from build123d import *

# Parameters (mm, degrees)
SKETCH1_W                       = 18
SKETCH1_H                       = 12
EXTRUDE1_DEPTH                  = 2
SKETCH2_W                       = 1.5
SKETCH2_H                       = 0.5
EXTRUDE2_DEPTH                  = 13
EXTRUDE3_DEPTH                  = 3
MIRROR2_COPY_1_DEPTH            = 3
SKETCH4_W                       = 6.5
SKETCH4_H                       = 12
EXTRUDE4_DEPTH                  = 5
SKETCH5_W                       = 1.5
SKETCH5_H                       = 0.8
EXTRUDE5_DEPTH                  = 13
F_2_56_TAPPED_HOLE1_D           = 1.778
F_2_56_TAPPED_HOLE1_DEPTH       = 9.4488
F_2_56_TAPPED_HOLE1_CBORE_D     = 2.1844
F_2_56_TAPPED_HOLE1_CBORE_DEPTH = 5.5372
F_2_56_TAPPED_HOLE1_TIP         = 0.53416509
SKETCH7_R                       = 1.5113
EXTRUDE6_DEPTH                  = 3.0226


with BuildPart() as part:
    # Sketch1 → Extrude1 (new body)
    with BuildSketch(Plane(origin=(0, 0, 0), x_dir=(1, 0, 0), z_dir=(0, 1, 0))):
        with Locations((-9, 6)):
            Rectangle(SKETCH1_W, SKETCH1_H)
    extrude(amount=-EXTRUDE1_DEPTH)

    # Sketch2 → Extrude2 (cut, through all)
    with BuildSketch(Plane.XY):
        with Locations((-9, -1.75)):
            Rectangle(SKETCH2_W, SKETCH2_H)
    extrude(amount=-EXTRUDE2_DEPTH, mode=Mode.SUBTRACT)

    # Sketch3 → Extrude3 (cut, through all)
    with BuildSketch(Plane(origin=(0, 0, 0), x_dir=(1, 0, 0), z_dir=(0, 1, 0))):
        with BuildLine():
            Line((-16.793731354, 2.5), (-16.793731354, 3.5))
            ThreePointArc((-16.793731354, 3.5), (-15.293731354, 5), (-13.793731354, 3.5))
            Line((-13.793731354, 3.5), (-13.793731354, 2.5))
            ThreePointArc((-13.793731354, 2.5), (-15.293731354, 1), (-16.793731354, 2.5))
        make_face()
    extrude3 = extrude(amount=-EXTRUDE3_DEPTH, mode=Mode.SUBTRACT)

    # Mirror1: Extrude3 across plane
    add(extrude3.mirror(Plane(origin=(0, 0, -6), x_dir=(1, 0, 0), z_dir=(0, 0, -1))), mode=Mode.SUBTRACT)

    # Mirror2: Extrude3 across plane
    add(extrude3.mirror(Plane(origin=(-9, 0, 0), x_dir=(0, 0, 1), z_dir=(1, 0, 0))), mode=Mode.SUBTRACT)

    # Mirror2 copy 1 sketch → Mirror2 copy 1 (cut, through all)
    with BuildSketch(Plane(origin=(-18, 0, -12), x_dir=(-1, 0, 0), z_dir=(0, 1, 0))):
        with BuildLine():
            Line((-16.793731354, 2.5), (-16.793731354, 3.5))
            ThreePointArc((-16.793731354, 3.5), (-15.293731354, 5), (-13.793731354, 3.5))
            Line((-13.793731354, 3.5), (-13.793731354, 2.5))
            ThreePointArc((-13.793731354, 2.5), (-15.293731354, 1), (-16.793731354, 2.5))
        make_face()
    extrude(amount=-MIRROR2_COPY_1_DEPTH, mode=Mode.SUBTRACT)

    # Sketch4 → Extrude4 (add)
    with BuildSketch(Plane(origin=(0, 0, 0), x_dir=(1, 0, 0), z_dir=(0, 1, 0))):
        with Locations((-8.75, 6)):
            Rectangle(SKETCH4_W, SKETCH4_H)
    extrude(amount=EXTRUDE4_DEPTH)

    # Sketch5 → Extrude5 (cut, through all)
    with BuildSketch(Plane.XY):
        with Locations((-11.25, 4.6)):
            Rectangle(SKETCH5_W, SKETCH5_H)
    extrude(amount=-EXTRUDE5_DEPTH, mode=Mode.SUBTRACT)

    # #2-56 Tapped Hole1
    with Locations(Plane(origin=(-8, 5, -2.6), x_dir=(0, 0, 1), z_dir=(0, 1, 0))):
        with Locations((0, 0), (-6.8, 0)):
            CounterBoreHole(F_2_56_TAPPED_HOLE1_D / 2, F_2_56_TAPPED_HOLE1_CBORE_D / 2, F_2_56_TAPPED_HOLE1_CBORE_DEPTH, depth=F_2_56_TAPPED_HOLE1_DEPTH)
            with Locations((0, 0, -(F_2_56_TAPPED_HOLE1_DEPTH + F_2_56_TAPPED_HOLE1_TIP / 2))):  # 118° drill point
                Cone(0, F_2_56_TAPPED_HOLE1_D / 2, F_2_56_TAPPED_HOLE1_TIP, mode=Mode.SUBTRACT)

    # Sketch7 → Extrude6 (cut)
    with BuildSketch(Plane.XY):
        with Locations((-9, 0.3)):
            Circle(SKETCH7_R)
    extrude6 = extrude(amount=-EXTRUDE6_DEPTH, mode=Mode.SUBTRACT)

    # Mirror3: Extrude6 across plane
    add(extrude6.mirror(Plane(origin=(0, 0, -6), x_dir=(1, 0, 0), z_dir=(0, 0, -1))), mode=Mode.SUBTRACT)


solid = part.part
Work out the finished part from the listing and answer in its coordinate system (mm). A direction names the side the tool comes from. Coordinates: 2 decimals unless noted, no trailing zeros. Order: outer loops, then holes, each group sorted by start corner. A loop starts at its lowest first (then second) coordinate and runs counter-clockwise, first axis right, second up. Notation, with made-up numbers: (43.25, 28) - (48.25, 28) arc R13 cw to (48.25, 43) - close; hole circle Ø4 at (84, 29.25). An arc over 180 degrees is marked (long way). Put each result on its own line as item: value. Start each with the question number.
1) For a pull along Z with two mould halves and no side action, classify faces 1 (the flat face through (-10, 0, -3.023)), 2 (the cylindrical face through (-7.12, -1.28, -9.28)), 3 (the flat face through (-14, -2, -6)) as released by +Z, released by -Z, zero draft, split by the parting line, or undercut.
2) Find the intervals of material crossed by line 1 (Z direction, x = -8, y = 3.1); line 2 (X direction, y = -1.25, z = -2.6); line 3 (Z direction, x = -14, y = -0.5), in increasing order. Write a range as from..to.
3) Find section A-A (z = -6.75). Give the vertices of the cut face in (x, y), plus the area to 4 significant figures.
4) Find section C-C (z = -2.25). Give the vertices of the cut face in (x, y), plus the area to 3 significant figures.
5) Find section B-B (y = 2.25). Give the vertices of the cut face in (x, z).
6) For faces 4 (the flat face through (-15, 0, -6)), 5 (the flat face through (-4.206, -1, -3)), 6 (the flat face through (-10, 0, -8.977)), 7 (the cylindrical face through (-7.262, 2.885, -3.405)), determine the directions among +Z, -Z, +X, -X, +Y, -Y from which every point of the face is accessible in a straight line to the end or side of a thin tool.
7) Flat-ended cylindrical pins translate along their axes: pin 1 (3 mm diameter, centred on x = -16.5, z = -5.5, fed in from +Y); pin 2 (1.1 mm diameter, centred on x = -8, z = -2.6, fed in from -Y); pin 3 (0.9 mm diameter, centred on y = 4.5, z = -4, fed in from -X); pin 4 (0.8 mm diameter, centred on x = -9, z = -8.5, fed in from -Y). Find the tip coordinate at first contact, or state that the pin passes through.
8) Find section D-D (x = -15.5). Give the vertices of the cut face in (y, z), plus the area to 3 significant figures.
Results list:
1. face 1: released by +Z
1. face 2: undercut
1. face 3: zero draft
2. line 1: z = -12..-10.49, -8.31..-3.69, -1.51..0
2. line 2: x = -18..-16.79, -13.79..-8.89, -7.11..-4.21, -1.21..0
2. line 3: z = -12..-10.26, -7.74..-4.26, -1.74..0
3. outline: (-18, -2) - (-9.75, -2) - (-9.75, -1.5) - (-8.25, -1.5) - (-8.25, -2) - (0, -2) - (0, 0) - (-5.5, 0) - (-5.5, 5) - (-10.5, 5) - (-10.5, 4.2) - (-12, 4.2) - (-12, 0) - (-18, 0) - close
3. area: 66.55 mm^2
4. outline: (-18, -2) - (-16.77, -2) - (-16.77, 0) - (-18, 0) - close; (-13.81, -2) - (-9.75, -2) - (-9.75, -1.5) - (-8.82, -1.5) - (-8.82, -1.2) arc R1.51 cw (long way) to (-9.03, 1.81) - (-9.03, 5) - (-10.5, 5) - (-10.5, 4.2) - (-12, 4.2) - (-12, 0) - (-13.81, 0) - close; (-7.18, -2) - (-4.19, -2) - (-4.19, 0) - (-5.5, 0) - (-5.5, 5) - (-6.97, 5) - (-6.97, -0.54) - (-7.18, -0.54) - close; (-1.23, -2) - (0, -2) - (0, 0) - (-1.23, 0) - close
4. area: 37.5 mm^2
5. outline: (-12, -12) - (-5.5, -12) - (-5.5, 0) - (-12, 0) - close; hole circle Ø2.18 at (-8, -9.4); hole circle Ø2.18 at (-8, -2.6)
6. face 4: +Z, -Z, -X, +Y
6. face 5: +Y, -Y
6. face 6: -Z
6. face 7: +Y
7. pin 1: stops at y = 0
7. pin 2: passes through
7. pin 3: stops at x = -12
7. pin 4: stops at y = -1.5
8. outline: (-2, -12) - (0, -12) - (0, -10.99) - (-2, -10.99) - close; (-2, -7.01) - (0, -7.01) - (0, -4.99) - (-2, -4.99) - close; (-2, -1.01) - (0, -1.01) - (0, 0) - (-2, 0) - close
8. area: 8.11 mm^2
